Part model, mm, in its own coordinate system. Give positions to 0.01 mm unless a question says otherwise; leave off trailing zeros. Write each loop counter-clockwise with the first axis right and the second up, starting at its lowest first coordinate (ties: lowest second). Pieces come first, ordered by that corner, then holes.
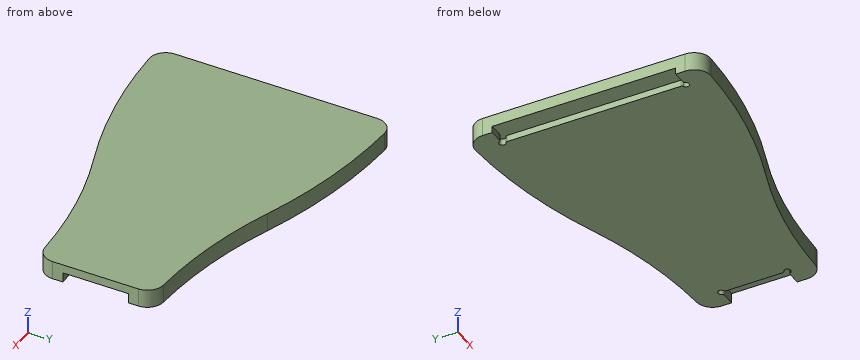
from build123d import *

# Parameters (mm, degrees)
F1_DEPTH = 28
F2_START = 10
F2_DEPTH = 18
F3_START = 15
F3_DEPTH = 13


with BuildPart() as f1:
    # F0 (on Top) → F1 (new body)
    with BuildSketch(Plane.XY):
        with BuildLine():
            ThreePointArc((475.8903838544, 90.4294724937), (368.2302608049, 102.9485734508), (263.9480821387, 132.489345215))
            ThreePointArc((263.9480821387, 132.489345215), (146.799756159, 165.6285981358), (25.853889943, 179.5583436206))
            ThreePointArc((25.853889943, 179.5583436206), (7.6268489987, 172.5499609003), (0, 154.5729304368))
            Line((0, 154.5729304368), (0, 140))
            Line((0, 140), (20.5838015129, 140))
            ThreePointArc((20.5838015129, 140), (22.260852496, 140.5125314072), (23.3648759456, 141.875))
            ThreePointArc((23.3648759456, 141.875), (31.5355339059, 143.5355339059), (29.875, 135.3648759456))
            ThreePointArc((29.875, 135.3648759456), (28.5125314072, 134.260852496), (28, 132.5838015129))
            Line((28, 132.5838015129), (28, 128.9779645573))
            Line((28, 128.9779645573), (28, -128.9779645573))
            Line((28, -128.9779645573), (28, -132.5838015129))
            ThreePointArc((28, -132.5838015129), (28.5125314072, -134.260852496), (29.875, -135.3648759456))
            ThreePointArc((29.875, -135.3648759456), (31.5355339059, -143.5355339059), (23.3648759456, -141.875))
            ThreePointArc((23.3648759456, -141.875), (22.260852496, -140.5125314072), (20.5838015129, -140))
            Line((20.5838015129, -140), (0, -140))
            Line((0, -140), (0, -154.5729304368))
            ThreePointArc((0, -154.5729304368), (7.6268489987, -172.5499609003), (25.853889943, -179.5583436206))
            ThreePointArc((25.853889943, -179.5583436206), (146.799756159, -165.6285981358), (263.9480821387, -132.489345215))
            ThreePointArc((263.9480821387, -132.489345215), (368.2302608049, -102.9485734508), (475.8903838544, -90.4294724937))
            ThreePointArc((475.8903838544, -90.4294724937), (492.989713677, -82.8053505266), (500, -65.445333193))
            Line((500, -65.445333193), (500, -50))
            ThreePointArc((500, -50), (489.712690089, -50.0738092009), (479.4274983284, -50.2952216062))
            ThreePointArc((479.4274983284, -50.2952216062), (477.7595252441, -50.8602066094), (476.6959890071, -52.2638564719))
            ThreePointArc((476.6959890071, -52.2638564719), (468.5248750874, -54.1419014019), (470.125, -45.9118494147))
            ThreePointArc((470.125, -45.9118494147), (471.4874685928, -44.8078259652), (472, -43.1307749821))
            Line((472, -43.1307749821), (472, -40.993877733))
            Line((472, -40.993877733), (472, 40.993877733))
            Line((472, 40.993877733), (472, 43.1307749821))
            ThreePointArc((472, 43.1307749821), (471.4874685928, 44.8078259652), (470.125, 45.9118494147))
            ThreePointArc((470.125, 45.9118494147), (468.5248750874, 54.1419014019), (476.6959890071, 52.2638564719))
            ThreePointArc((476.6959890071, 52.2638564719), (477.7595252441, 50.8602066094), (479.4274983284, 50.2952216062))
            ThreePointArc((479.4274983284, 50.2952216062), (489.712690089, 50.0738092009), (500, 50))
            Line((500, 50), (500, 65.445333193))
            ThreePointArc((500, 65.445333193), (492.989713677, 82.8053505266), (475.8903838544, 90.4294724937))
        make_face()
    extrude(amount=F1_DEPTH)

    # F0 (on Top) → F2 (join)
    with BuildSketch(Plane.XY.offset(F2_START)):
        with BuildLine():
            Line((20.5838015129, 140), (0, 140))
            Line((0, 140), (0, -140))
            Line((0, -140), (20.5838015129, -140))
            ThreePointArc((20.5838015129, -140), (22.260852496, -140.5125314072), (23.3648759456, -141.875))
            ThreePointArc((23.3648759456, -141.875), (31.5355339059, -143.5355339059), (29.875, -135.3648759456))
            ThreePointArc((29.875, -135.3648759456), (28.5125314072, -134.260852496), (28, -132.5838015129))
            Line((28, -132.5838015129), (28, -128.9779645573))
            Line((28, -128.9779645573), (28, 128.9779645573))
            Line((28, 128.9779645573), (28, 132.5838015129))
            ThreePointArc((28, 132.5838015129), (28.5125314072, 134.260852496), (29.875, 135.3648759456))
            ThreePointArc((29.875, 135.3648759456), (31.5355339059, 143.5355339059), (23.3648759456, 141.875))
            ThreePointArc((23.3648759456, 141.875), (22.260852496, 140.5125314072), (20.5838015129, 140))
        make_face()
    extrude(amount=F2_DEPTH)

    # F0 (on Top) → F3 (join)
    with BuildSketch(Plane.XY.offset(F3_START)):
        with BuildLine():
            Line((500, -50), (500, 50))
            ThreePointArc((500, 50), (489.712690089, 50.0738092009), (479.4274983284, 50.2952216062))
            ThreePointArc((479.4274983284, 50.2952216062), (477.7595252441, 50.8602066094), (476.6959890071, 52.2638564719))
            ThreePointArc((476.6959890071, 52.2638564719), (468.5248750874, 54.1419014019), (470.125, 45.9118494147))
            ThreePointArc((470.125, 45.9118494147), (471.4874685928, 44.8078259652), (472, 43.1307749821))
            Line((472, 43.1307749821), (472, 40.993877733))
            Line((472, 40.993877733), (472, -40.993877733))
            Line((472, -40.993877733), (472, -43.1307749821))
            ThreePointArc((472, -43.1307749821), (471.4874685928, -44.8078259652), (470.125, -45.9118494147))
            ThreePointArc((470.125, -45.9118494147), (468.5248750874, -54.1419014019), (476.6959890071, -52.2638564719))
            ThreePointArc((476.6959890071, -52.2638564719), (477.7595252441, -50.8602066094), (479.4274983284, -50.2952216062))
            ThreePointArc((479.4274983284, -50.2952216062), (489.712690089, -50.0738092009), (500, -50))
        make_face()
    extrude(amount=F3_DEPTH)


solid = f1.part
1) Flat gauge pins, fed straight in: P1, Ø10, axis at x = 17, y = -51, coming from the -Z side; P2, Ø4.5, axis at y = 6, z = 7.5, coming from the +X side; P3, Ø6, axis at y = -85, z = 21.5, coming from the +X side. Where does each tip first touch, or does it go through?
Check result:
P1: stops at z = 10
P2: stops at x = 472
P3: stops at x = 493.73
2) Drill centre lines: L1, parallel to X at y = 39, z = 7.5; L2, parallel to Y at x = 339.5, z = 1.75; L3, parallel to Y at x = 115.5, z = 20. Where is each one in solid material? Low to high.
Check result:
L1: x = 28 to 472
L2: y = -109.3 to 109.3
L3: y = -171.14 to 171.14
3) Saw through at B-B (z = 21.5). Write the cut outline in (x, y), and give its area (3 significant figures).
Check result:
outline: (0, -154.57) arc R25 ccw to (25.85, -179.56) arc R756.94 ccw to (263.95, -132.49) arc R676.94 cw to (475.89, -90.43) arc R25 ccw to (500, -65.45) - (500, 65.45) arc R25 ccw to (475.89, 90.43) arc R676.94 cw to (263.95, 132.49) arc R756.94 ccw to (25.85, 179.56) arc R25 ccw to (0, 154.57) - close
area: 135,000 mm2
4) Saw through at C-C (x = 420). Write the cut outline in (y, z).
Check result:
outline: (-94.74, 0) - (94.74, 0) - (94.74, 28) - (-94.74, 28) - close
5) Saw through at D-D (y = -82). Write the cut outline in (x, z).
Check result:
outline: (0, 10) - (28, 10) - (28, 0) - (493.73, 0) - (493.73, 28) - (0, 28) - close
6) Saw through at A-A (y = -27). Write the cut outline in (x, z), and give its area (3 significant figures).
Check result:
outline: (0, 10) - (28, 10) - (28, 0) - (472, 0) - (472, 15) - (500, 15) - (500, 28) - (0, 28) - close
area: 13,300 mm2
